Here's how the part is built. I have some questions about the finished solid (model axes, mm). A direction names the side the tool comes from. Round coordinates to 2 decimals unless told otherwise and drop trailing zeros. Answer in a Markdown table with one row per item.
from build123d import *

# Parameters (mm, degrees)
SKETCH3_W           = 21.993363762
SKETCH3_H           = 30.202832843
CUT_EXTRUDE1_DEPTH  = 100
SKETCH5_R           = 3.75
CUT_EXTRUDE4_DEPTH  = 15.5
SKETCH6_R           = 6.9
CUT_EXTRUDE5_DEPTH  = 22
SKETCH7_R           = 1.2
CUT_EXTRUDE6_DEPTH  = 6.2
SKETCH8_R           = 12.5
CUT_EXTRUDE7_DEPTH  = 4.8
SKETCH9_R           = 9.25
CUT_EXTRUDE8_DEPTH  = 21.6
SKETCH10_R          = 1.71
CUT_EXTRUDE9_DEPTH  = 40
SKETCH12_W          = 0.5
SKETCH12_H          = 24.9
CUT_EXTRUDE10_DEPTH = 2
SKETCH13_W          = 0.5
SKETCH13_H          = 21.6
CUT_EXTRUDE11_DEPTH = 10
SKETCH14_W          = 0.5
SKETCH14_H          = 4.8
CUT_EXTRUDE12_DEPTH = 12.5
SKETCH15_W          = 0.5
SKETCH15_H          = 6.2
CUT_EXTRUDE13_DEPTH = 1.5
SKETCH16_W          = 0.500221157
SKETCH16_H          = 22
CUT_EXTRUDE14_DEPTH = 7
SKETCH17_W          = 0.505614017
SKETCH17_H          = 15.5
CUT_EXTRUDE15_DEPTH = 4
CUT_EXTRUDE16_START = -1
SKETCH18_R          = 3
CUT_EXTRUDE16_DEPTH = 15


with BuildPart() as part:
    # Loft1: read off the stored shape, not the designer's step
    # Loft1: loft between two sections, ruled curve by curve
    loft1_from = [
        Edge.make_bspline([(-4.381363328, 0, -14.084252035), (-32.549867398, 0, -5.321525378), (-23.787140742, 0, 22.846978692), (4.381363328, 0, 14.084252035), (32.549867398, 0, 5.321525378), (23.787140742, 0, -22.846978692), (-4.381363328, 0, -14.084252035)], [0, 0, 0, 0, 0.5, 0.5, 0.5, 1, 1, 1, 1], 3, [1, 0.333333333, 0.333333333, 1, 0.333333333, 0.333333333, 1]),
    ]
    loft1_to = [
        Edge.make_bspline([(-7.165507724, 95, -13.092407115), (-33.350321953, 95, 1.238608334), (-19.019306505, 95, 27.423422563), (7.165507724, 95, 13.092407115), (33.350321953, 95, -1.238608334), (19.019306505, 95, -27.423422563), (-7.165507724, 95, -13.092407115)], [0, 0, 0, 0, 0.5, 0.5, 0.5, 1, 1, 1, 1], 3, [1, 0.333333333, 0.333333333, 1, 0.333333333, 0.333333333, 1]),
    ]
    loft1 = Solid(Shell([*[Face.make_surface_from_curves(loft1_from[k], loft1_to[k]) for k in range(1)], Face(Wire(loft1_from)), Face(Wire(loft1_to))]))
    add(loft1)

    # Sketch3 → Cut-Extrude1 (cut)
    with BuildSketch(Plane(origin=(0, 0, 0), x_dir=(1, 0, 0), z_dir=(0, 1, 0))):
        with Locations((10.996681881, -0.176416421)):
            Rectangle(SKETCH3_W, SKETCH3_H)
    extrude(amount=CUT_EXTRUDE1_DEPTH, mode=Mode.SUBTRACT)

    # Sketch5 → Cut-Extrude4 (cut)
    with BuildSketch(Plane(origin=(0, 0, 0), x_dir=(1, 0, 0), z_dir=(0, 1, 0))):
        Circle(SKETCH5_R)
    extrude(amount=CUT_EXTRUDE4_DEPTH, mode=Mode.SUBTRACT)

    # Sketch6 → Cut-Extrude5 (cut)
    with BuildSketch(Plane(origin=(0, 15.5, 0), x_dir=(-1, 0, 0), z_dir=(0, -1, 0))):
        Circle(SKETCH6_R)
    extrude(amount=-CUT_EXTRUDE5_DEPTH, mode=Mode.SUBTRACT)

    # Sketch7 → Cut-Extrude6 (cut)
    with BuildSketch(Plane(origin=(0, 37.5, 0), x_dir=(-1, 0, 0), z_dir=(0, -1, 0))):
        Circle(SKETCH7_R)
    extrude(amount=-CUT_EXTRUDE6_DEPTH, mode=Mode.SUBTRACT)

    # Sketch8 → Cut-Extrude7 (cut)
    with BuildSketch(Plane(origin=(0, 43.7, 0), x_dir=(-1, 0, 0), z_dir=(0, -1, 0))):
        Circle(SKETCH8_R)
    extrude(amount=-CUT_EXTRUDE7_DEPTH, mode=Mode.SUBTRACT)

    # Sketch9 → Cut-Extrude8 (cut)
    with BuildSketch(Plane(origin=(0, 48.5, 0), x_dir=(-1, 0, 0), z_dir=(0, -1, 0))):
        Circle(SKETCH9_R)
    extrude(amount=-CUT_EXTRUDE8_DEPTH, mode=Mode.SUBTRACT)

    # Sketch10 → Cut-Extrude9 (cut)
    with BuildSketch(Plane(origin=(0, 95, 0), x_dir=(1, 0, 0), z_dir=(0, 1, 0))):
        Circle(SKETCH10_R)
    extrude(amount=-CUT_EXTRUDE9_DEPTH, mode=Mode.SUBTRACT)

    # Sketch12 → Cut-Extrude10 (cut)
    with BuildSketch(Plane(origin=(0, 0, 0), x_dir=(0, 0, -1), z_dir=(1, 0, 0))):
        with Locations((0, 82.55)):
            Rectangle(SKETCH12_W, SKETCH12_H)
    extrude(amount=-CUT_EXTRUDE10_DEPTH, mode=Mode.SUBTRACT)

    # Sketch13 → Cut-Extrude11 (cut)
    with BuildSketch(Plane(origin=(0, 0, 0), x_dir=(0, 0, -1), z_dir=(1, 0, 0))):
        with Locations((0, 59.3)):
            Rectangle(SKETCH13_W, SKETCH13_H)
    extrude(amount=-CUT_EXTRUDE11_DEPTH, mode=Mode.SUBTRACT)

    # Sketch14 → Cut-Extrude12 (cut)
    with BuildSketch(Plane(origin=(0, 0, 0), x_dir=(0, 0, -1), z_dir=(1, 0, 0))):
        with Locations((0, 46.1)):
            Rectangle(SKETCH14_W, SKETCH14_H)
    extrude(amount=-CUT_EXTRUDE12_DEPTH, mode=Mode.SUBTRACT)

    # Sketch15 → Cut-Extrude13 (cut)
    with BuildSketch(Plane(origin=(0, 0, 0), x_dir=(0, 0, -1), z_dir=(1, 0, 0))):
        with Locations((0, 40.6)):
            Rectangle(SKETCH15_W, SKETCH15_H)
    extrude(amount=-CUT_EXTRUDE13_DEPTH, mode=Mode.SUBTRACT)

    # Sketch16 → Cut-Extrude14 (cut)
    with BuildSketch(Plane(origin=(0, 0, 0), x_dir=(0, 0, -1), z_dir=(1, 0, 0))):
        with Locations((0.000110579, 26.5)):
            Rectangle(SKETCH16_W, SKETCH16_H)
    extrude(amount=-CUT_EXTRUDE14_DEPTH, mode=Mode.SUBTRACT)

    # Sketch17 → Cut-Extrude15 (cut)
    with BuildSketch(Plane(origin=(0, 0, 0), x_dir=(0, 0, -1), z_dir=(1, 0, 0))):
        with Locations((-0.002585851, 7.75)):
            Rectangle(SKETCH17_W, SKETCH17_H)
    extrude(amount=-CUT_EXTRUDE15_DEPTH, mode=Mode.SUBTRACT)

    # Sketch18 → Cut-Extrude16 (cut)
    with BuildSketch(Plane(origin=(0, 0, 0), x_dir=(0, 0, -1), z_dir=(1, 0, 0)).offset(CUT_EXTRUDE16_START)):
        with Locations((-9.326204078, 6.12452291)):
            Circle(SKETCH18_R)
        with Locations((-9.25, 84.904010386)):
            Circle(SKETCH18_R)
        with Locations((9.326204078, 6.12452291)):
            Circle(SKETCH18_R)
        with Locations((9.25, 84.904010386)):
            Circle(SKETCH18_R)
    extrude(amount=-CUT_EXTRUDE16_DEPTH, mode=Mode.SUBTRACT)


solid = part.part
1) We'd pull the mould along Z, two halves only. Please class faces 1 (the face through (-4.843, 26.346, -4.915)), 2 (the face through (0, 47, 13)): +Z half, -Z half, draft (parallel to the pull), parting line (faces both ways), or undercut.
Response:
| item | result |
|---|---|
| face 1 | undercut |
| face 2 | draft |
2) For pin 1 (3 mm diameter, centred on x = -2, y = 62, fed in from +Z); pin 2 (3 mm diameter, centred on y = 85, z = -9, fed in from -X); pin 3 (4 mm diameter, centred on x = -2, y = 45.5, fed in from -Z), each with a flat end and sliding along its axis, tell me the tip position at first contact or that it passes through.
Response:
| item | result |
|---|---|
| pin 1 | stops at z = 14.79 |
| pin 2 | stops at x = -1 |
| pin 3 | stops at z = -14.76 |
3) I need wall thicknesses on line 1 (Y direction, x = -7, z = 3.25); line 2 (Z direction, x = -7.75, y = 7.5); line 3 (Y direction, x = -8.5, z = -9.25). Which ranges of each line are inside material? Lowest first, please. Write a range as [from, to].
Response:
| item | result |
|---|---|
| line 1 | y = [0, 43.7], [70.1, 95] |
| line 2 | z = [-12.54, -11.99], [-6.66, 6.66], [11.99, 12.54] |
| line 3 | y = [0, 3.13], [9.12, 81.9], [87.9, 95] |
4) Which directions (+Z, -Z, +X, -X, +Y, -Y) give clear straight access to the entire face, cutting with the end or side of a thin tool? Please do faces 3 (the face through (-4, 70.1, 0)), 4 (the face through (-1, 85, -9)), 5 (the face through (0, 47, -13)).
Response:
| item | result |
|---|---|
| face 3 | +X |
| face 4 | -X |
| face 5 | +Z, -Z, +X, +Y, -Y |
5) I want a section at A-A, the plane x = -5.75. Count the separate pieces of the cut face and the enclosed holes in it, and give its area (3 significant figures).
Response:
| item | result |
|---|---|
| separate pieces | 1 |
| enclosed holes | 6 |
| area | 1,890 mm^2 |
